from build123d import *

# Parameters (mm, degrees)
F0_W      = 5
F0_H      = 15
F1_DEPTH  = 20
F3_DEPTH  = 5
F2_W      = 10
F2_H      = 10
F4_DEPTH  = 20.001
F6_DEPTH  = 5
F5_R      = 5
F7_DEPTH  = 5
F8_R      = 5.5
F8_R_2    = 5
F9_DEPTH  = 2.5
F11_R     = 3.5
F9_FACE_R = 5.5


with BuildPart() as f1:
    # F0 (on Front) → F1 (new body)
    with BuildSketch(Plane.XZ):
        with BuildLine():
            ThreePointArc((7.5, -125), (3.9644660941, -123.5355339059), (2.5, -120))
            Line((2.5, -120), (-2.5, -120))
            ThreePointArc((-2.5, -120), (-1.6143782777, -124.1143782777), (0.8856217223, -127.5))
            ThreePointArc((0.8856217223, -127.5), (3.9644660941, -125.6458565331), (7.5, -125))
        make_face()
        with BuildLine():
            Line((-2.5, -120), (2.5, -120))
            Line((2.5, -120), (2.5, -111.3397459622))
            ThreePointArc((2.5, -111.3397459622), (-1.1602540378, -115), (-2.5, -120))
        make_face()
        with BuildLine():
            Line((-2.5, 120), (-2.5, -120))
            ThreePointArc((-2.5, -120), (-1.1602540378, -115), (2.5, -111.3397459622))
            Line((2.5, -111.3397459622), (2.5, 120))
            Line((2.5, 120), (-2.5, 120))
        make_face()
        with BuildLine():
            ThreePointArc((17.5, -135), (14.5710678119, -127.9289321881), (7.5, -125))
            Line((7.5, -125), (7.5, -130))
            ThreePointArc((7.5, -130), (11.0355339059, -131.4644660941), (12.5, -135))
            Line((12.5, -135), (17.5, -135))
        make_face()
        with BuildLine():
            Line((7.5, -130), (7.5, -125))
            ThreePointArc((7.5, -125), (3.9644660941, -125.6458565331), (0.8856217223, -127.5))
            ThreePointArc((0.8856217223, -127.5), (3.9644660941, -129.3541434669), (7.5, -130))
        make_face()
        with Locations((15, -142.5)):
            Rectangle(F0_W, F0_H)
    extrude(amount=F1_DEPTH)

    # F2 (on face) → F3 (join)
    with BuildSketch(Plane.YZ.offset(17.5)):
        with BuildLine():
            Line((0, -150), (-20, -150))
            ThreePointArc((-20, -150), (-10, -153), (0, -150))
        make_face()
    extrude(amount=-F3_DEPTH)

    # F2 (on face) → F4 (cut, through all)
    with BuildSketch(Plane.YZ.offset(17.5)):
        with Locations((-10, -142)):
            Rectangle(F2_W, F2_H)
    extrude(amount=-F4_DEPTH, mode=Mode.SUBTRACT)

    # F5 (on face) → F6 (join)
    with BuildSketch(Plane(origin=(-2.5, 0, 0), x_dir=(0, -1, 0), z_dir=(-1, 0, 0))):
        with BuildLine():
            Line((0, 120), (20, 120))
            ThreePointArc((20, 120), (10, 123), (0, 120))
        make_face()
    extrude(amount=-F6_DEPTH)

    # F5 (on face) → F7 (join)
    with BuildSketch(Plane(origin=(-2.5, 0, 0), x_dir=(0, -1, 0), z_dir=(-1, 0, 0))):
        with Locations((10, 114)):
            Circle(F5_R)
    extrude(amount=F7_DEPTH)

    # F8 (on face) → F9 (join)
    with BuildSketch(Plane(origin=(-7.5, 0, 0), x_dir=(0, -1, 0), z_dir=(-1, 0, 0))):
        with Locations((10, 114)):
            Circle(F8_R)
        with Locations((10, 114)):
            Circle(F8_R_2, mode=Mode.SUBTRACT)
        with Locations((10, 114)):
            Circle(F8_R_2)
    extrude(amount=F9_DEPTH)

    # F11 (on offset) → F12 section 0
    with BuildSketch(Plane(origin=(-14.5, 0, 0), x_dir=(0, -1, 0), z_dir=(-1, 0, 0))):
        with Locations((10, 114)):
            Circle(F11_R)
    # F9_face (on face) → F12 section 1
    with BuildSketch(Plane(origin=(-10, -10, 114), x_dir=(0, -1, 0), z_dir=(-1, 0, 0))):
        Circle(F9_FACE_R)
    loft()


solid = f1.part
Can you work these out from the model? Positions are in its coordinate system, mm. A direction names the side the tool comes from. Coordinates: 2 decimals unless noted, no trailing zeros. Order: outer loops, then holes, each group sorted by start corner. A loop starts at its lowest first (then second) coordinate and runs counter-clockwise, first axis right, second up. Notation, with made-up numbers: (18, 9) -> (33, 9) arc R6 ccw to (33, 16) -> close; hole circle Ø5 at (-22.5, 57.5). An arc over 180 degrees is marked (long way). Use one line per item in the form item = value.
Q1. Will these pins go through, and if not, where does the flat tip stop? P1, Ø5, axis at y = -2.5, z = -6, coming from the +X side; P2, Ø4, axis at y = -6.5, z = -57.5, coming from the -X side; P3, Ø4, axis at x = 14.5, y = -8.5, coming from the +Z side.
From the geometry:
P1 = 2.5
P2 = -2.5
P3 = -126.34
Q2. Imagine slicing it at B-B, the plane z = -11. List the corners of the cut face in (x, y) for me.
From the geometry:
outline = (-2.5, -20) -> (2.5, -20) -> (2.5, 0) -> (-2.5, 0) -> close
Q3. Imagine slicing it at A-A, the plane y = -10. List the corners of the cut face in (x, z) for me.
From the geometry:
outline = (-14.5, 110.5) -> (-10, 108.5) -> (-7.5, 108.5) -> (-7.5, 109) -> (-2.5, 109) -> (-2.5, -120) arc R10 ccw to (7.5, -130) arc R5 cw to (12.5, -135) -> (12.5, -137) -> (17.5, -137) -> (17.5, -135) arc R10 ccw to (7.5, -125) arc R5 cw to (2.5, -120) -> (2.5, 123) -> (-2.5, 123) -> (-2.5, 119) -> (-7.5, 119) -> (-7.5, 119.5) -> (-10, 119.5) -> (-14.5, 117.5) -> close; (12.5, -153) -> (17.5, -153) -> (17.5, -147) -> (12.5, -147) -> close
Q4. I need wall thicknesses on L1, parallel to X at y = -12, z = 78; L2, parallel to Z at x = 7, y = -18; L3, parallel to Z at x = -9, y = -10.75. Which ranges of each line are inside material? Lowest first, please.
From the geometry:
L1 = -2.5 to 2.5
L2 = -129.99 to -124.97
L3 = 108.55 to 119.45
Q5. We'd pull the mould along Y, two halves only. Please class faces 1 (the face through (4, -9.86, -123.57)), 2 (the face through (15, -10, -153)), 3 (the face through (15, -10, -137)), 4 (the face through (15, -15, -142)): released by +Y, released by -Y, zero draft, split by the parting line, or undercut.
From the geometry:
face_1 = zero draft
face_2 = split by the parting line
face_3 = undercut
face_4 = undercut
Q6. Which directions (+Z, -Z, +X, -X, +Y, -Y) give clear straight access to the entire face, cutting with the end or side of a thin tool? Please do faces 5 (the face through (2.5, -10, 3)), 6 (the face through (-8.732, -9.284, 119.453)), 7 (the face through (-7.5, -11.6, 109.1)).
From the geometry:
face_5 = +Z, +X, +Y, -Y
face_6 = -X
face_7 = none
